Geometry check sheet. Reference: the model listing, model coordinates, mm. A direction names the side the tool comes from. Round coordinates to 2 decimals unless told otherwise and drop trailing zeros. Order: outer loops, then holes, each group sorted by start corner. A loop starts at its lowest first (then second) coordinate and runs counter-clockwise, first axis right, second up. Notation, with made-up numbers: (24, -31) - (38, -31) arc R33 cw to (38, 4) - close; hole circle Ø7 at (-33.75, 44). An arc over 180 degrees is marked (long way). Use a Markdown table: item, result. Add a question column.
(1) Thickness scan on line 1 along X through (y, z) = (1.9, -6.25); line 2 along X through (y, z) = (2.8, 4.25); line 3 along X through (y, z) = (0.9, 11.5). Record the ranges inside material, lowest first. Write a range as [from, to].
(2) Section check C-C on x = 2. Record the boundary of the cut face in (y, z).
(3) Gauge pin test, flat ends, axial feed: P1, Ø2.5, axis at x = -1, z = 12.5, coming from the -Y side; P2, Ø2.5, axis at x = -11.1, z = -11.1, coming from the -Y side; P3, Ø0.6, axis at y = 0.5, z = -13, coming from the +X side. Record the tip position at first contact, or that the pin passes through.
(4) Mould release check, pull along X, two halves, no side actions. Record for faces 1 (the face through (-3, 1, 14)), 2 (the face through (-11.83, 1.479, -11.783)), 3 (the face through (13.43, 1.52, -13.4)): released by +X, released by -X, zero draft, split by the parting line, or undercut.
(5) Access from +Z, -Z, +X, -X, +Y, -Y to the whole of each face (thin tool, end or side, straight path). Record for faces 4 (the face through (12, 0, 0)), 5 (the face through (-11.1, 1, 0)), 6 (the face through (0, 0.5, -13)).
(6) Section check A-A on y = 1. Record the boundary of the cut face in (x, z), then the cut area to 3 significant figures.
(7) Section check B-B on z = 1. Record the boundary of the cut face in (x, y).
Autodesk Inventor part; units mm, degrees
ref_plane "YZ Plane" through (0, 0, 0) normal (1, 0, 0) x (0, 1, 0)
ref_plane "XZ Plane" through (0, 0, 0) normal (0, 1, 0) x (-1, 0, 0)
ref_plane "XY Plane" through (0, 0, 0) normal (0, 0, 1) x (1, 0, 0)
sketch "Sketch1" plane through (0, 0, 0) normal (0, 1, 0) x (-1, 0, 0)
  line L0 (-11.1, -11.1) -> (-10.1, -11.1)
  line L1 (11.1, -11.1) -> (11.1, -10.1)
  line L2 (11.1, 11.1) -> (10.1, 11.1)
  line L3 (-11.1, 11.1) -> (-11.1, 10.1)
  line L4 (-11.1, -11.1) -> (11.1, 11.1) construction
  line L5 (11.1, -11.1) -> (-11.1, 11.1) construction
  line L6 (-14, -14) -> (14, -14)
  line L7 (14, -14) -> (14, 14)
  line L8 (14, 14) -> (-14, 14)
  line L9 (-14, 14) -> (-14, -14)
  line L10 (-14, -14) -> (14, 14) construction
  line L11 (14, -14) -> (-14, 14) construction
  line L12 (14, 14) -> (20, 14)
  line L13 (20, 14) -> (20, -14)
  line L14 (20, -14) -> (14, -14)
  line L15 (14, -14) -> (14, 14)
  line L16 (3.6361, 0) -> (-5.9421, 0)
  circle A0 centre (11.1, 11.1) radius 1
  line L17 (0, 4.2823) -> (0, -4.7782)
  circle A1 centre (11.1, -11.1) radius 1
  circle A2 centre (-11.1, 11.1) radius 1
  circle A3 centre (-11.1, -11.1) radius 1
  line L18 (11.1, 10.1) -> (11.1, 11.1)
  line L19 (10.1, 11.1) -> (-10.1, 11.1)
  line L20 (11.1, -10.1) -> (11.1, 10.1)
  line L21 (10.1, -11.1) -> (11.1, -11.1)
  line L22 (-11.1, 10.1) -> (-11.1, -10.1)
  line L23 (-10.1, 11.1) -> (-11.1, 11.1)
  line L24 (-10.1, -11.1) -> (10.1, -11.1)
  line L25 (-11.1, -10.1) -> (-11.1, -11.1)
  point P0 (0, 0)
  point P1 (17, 6.25)
  point P2 (17, -6.25)
  dimension "d0" = 22.2
  dimension "d1" = 22.2
  dimension "d2" = 28
  dimension "d3" = 28
  dimension "d4" = 6
  dimension "d5" = 12.5
  dimension "d6" = 2
  dimension "d9" = 22.2
  dimension "d12" = 22.2
  dimension "d17" = 3
extrude "Extrusion1" add sketch "Sketch1" along normal blind 3
hole "Hole1" at (-17, 0, 6.25) at (-17, 0, -6.25) direction (0, 1, 0) diameter 3.1 end through all countersink diameter 6 countersink angle 90
fillet "Fillet1" radius 2 2 edges at (14, 1.5, -14) (14, 1.5, 14)
fillet "Fillet2" radius 2 2 edges at (-20, 1.5, -14) (-20, 1.5, 14)
sketch "Sketch2" plane through (0, 0, 0) normal (0, -1, 0) x (1, 0, 0)
  line L0 (12, -14) -> (-18, -14)
  line L1 (-9.5, 14) -> (9.5, 14)
  line L2 (9.5, 14) -> (9.5, -14)
  line L3 (9.5, -14) -> (-9.5, -14)
  line L4 (-9.5, -14) -> (-9.5, 14)
  line L5 (-9.5, 14) -> (9.5, -14) construction
  line L6 (9.5, 14) -> (-9.5, -14) construction
  point P0 (0, 0)
  dimension "d27" = 19
extrude "Extrusion2" cut sketch "Sketch2" against normal blind 0.5
properties part number "Metal_mount_horizontal_coverslip22x22_v2"
Check sheet entries:
| question | item | result |
|---|---|---|
| 1 | line 1 | x = [-20, -18.55], [-15.45, -11.1], [11.1, 14] |
| 1 | line 2 | x = [-20, -11.1], [11.1, 14] |
| 1 | line 3 | x = [-20, -12.02], [-10.18, 10.18], [12.02, 14] |
| 2 | outline | (0.5, -14) - (3, -14) - (3, -11.1) - (0.5, -11.1) - close; (0.5, 11.1) - (3, 11.1) - (3, 14) - (0.5, 14) - close |
| 3 | P1 | stops at y = 0.5 |
| 3 | P2 | stops at y = 0 |
| 3 | P3 | stops at x = 13.87 |
| 4 | face 1 | zero draft |
| 4 | face 2 | undercut |
| 4 | face 3 | released by +X |
| 5 | face 4 | +Z, -Z, +X, -X, -Y |
| 5 | face 5 | +Y, -Y |
| 5 | face 6 | +Z, -Z, -Y |
| 6 | outline | (-20, -12) arc R2 ccw to (-18, -14) - (12, -14) arc R2 ccw to (14, -12) - (14, 12) arc R2 ccw to (12, 14) - (-18, 14) arc R2 ccw to (-20, 12) - close; hole circle Ø4 at (-17, -6.25); hole circle Ø4 at (-17, 6.25); hole (-11.1, -10.1) arc R1 ccw (long way) to (-10.1, -11.1) - (10.1, -11.1) arc R1 ccw (long way) to (11.1, -10.1) - (11.1, 10.1) arc R1 ccw (long way) to (10.1, 11.1) - (-10.1, 11.1) arc R1 ccw (long way) to (-11.1, 10.1) - close |
| 6 | area | 421 mm2 |
| 7 | outline | (-20, 0) - (-11.1, 0) - (-11.1, 3) - (-20, 3) - close; (11.1, 0) - (14, 0) - (14, 3) - (11.1, 3) - close |
